```python
from build123d import *

# Parameters (mm, degrees)
BOSS_EXTRUDE1_DEPTH            = 60
CBORE_FOR_M3_SHCS1_D           = 3.4
CBORE_FOR_M3_SHCS1_DEPTH       = 5
CBORE_FOR_M3_SHCS1_CBORE_D     = 6.5
CBORE_FOR_M3_SHCS1_CBORE_DEPTH = 3
CBORE_FOR_M3_SHCS1_TIP         = 1.021463052


with BuildPart() as part:
    # Sketch3 → Boss-Extrude1 (new body)
    with BuildSketch(Plane.XY):
        Polygon((0, 60.2), (0, 33.96), (-3, 35.94), (-3, 55.2), (-12, 55.2), (-12, 60.2), align=None)
    extrude(amount=BOSS_EXTRUDE1_DEPTH)

    # CBORE for M3 SHCS1
    with Locations(Plane(origin=(0, 60.2, 0), x_dir=(1, 0, 0), z_dir=(0, 1, 0))):
        with Locations((-7.5, -15), (-7.5, -45)):
            CounterBoreHole(CBORE_FOR_M3_SHCS1_D / 2, CBORE_FOR_M3_SHCS1_CBORE_D / 2, CBORE_FOR_M3_SHCS1_CBORE_DEPTH, depth=CBORE_FOR_M3_SHCS1_DEPTH)
            with Locations((0, 0, -(CBORE_FOR_M3_SHCS1_DEPTH + CBORE_FOR_M3_SHCS1_TIP / 2))):  # 118° drill point
                Cone(0, CBORE_FOR_M3_SHCS1_D / 2, CBORE_FOR_M3_SHCS1_TIP, mode=Mode.SUBTRACT)


solid = part.part
```
Verification items for the finished model (mm, model axes). A direction names the side the tool comes from. Coordinates: 2 decimals unless noted, no trailing zeros. Loops run counter-clockwise (first coordinate to the right, second up) from the corner with the lowest first, then second, coordinate; pieces in that order, holes last. Notation, with made-up numbers: (6, 78) -> (42, 78) arc R31 ccw to (42, 111) -> close; hole circle Ø6 at (-18.5, 48). An arc over 180 degrees is marked (long way). Answer in a Markdown table with one row per item. Add a question column.
1. Section check A-A, the plane x = -7.5. Enter the section's corners in (y, z).
2. Depth check by flat-ended pin: P1, Ø1, axis at y = 40.5, z = 17, coming from the -X side; P2, Ø6, axis at x = -7.5, z = 45, coming from the +Y side; P3, Ø4, axis at x = -7.5, z = 15, coming from the -Y side. Enter the tip coordinate at first touch or a pass-through.
3. Access from +Z, -Z, +X, -X, +Y, -Y to the whole of each face (thin tool, end or side, straight path). Record for faces 1 (the face through (-6, 60.2, 30)), 2 (the face through (-6.1, 57.2, 16.4)), 3 (the face through (-7, 55.2, 30)).
4. Draft check along Z on faces 4 (the face through (-2, 53, 0)), 5 (the face through (-12, 58, 30)), 6 (the face through (-5.8, 56.19, 14.93)). Enter one of: +Z half, -Z half, draft (parallel to the pull), parting line (faces both ways), or undercut.
5. Section check D-D, the plane x = -1. Enter the section's corners in (y, z), then the cut area to 3 significant figures.
6. Material ranges on probe 1 along Z at (x, y) = (-7.5, 59.5); probe 2 along Z at (x, y) = (-7.5, 56.3); probe 3 along X at (y, z) = (55.65, 45), recorded low to high. Write a range as [from, to].
7. Section check C-C, the plane z = 36. Enter the section's corners in (x, y), then the cut area to 3 significant figures.
8. Section check B-B, the plane z = 45. Enter the section's corners in (x, y).
Derived:
| question | item | result |
|---|---|---|
| 1 | outline | (55.2, 0) -> (60.2, 0) -> (60.2, 11.75) -> (57.2, 11.75) -> (57.2, 13.3) -> (55.2, 13.3) -> close; (55.2, 16.7) -> (57.2, 16.7) -> (57.2, 18.25) -> (60.2, 18.25) -> (60.2, 41.75) -> (57.2, 41.75) -> (57.2, 43.3) -> (55.2, 43.3) -> close; (55.2, 46.7) -> (57.2, 46.7) -> (57.2, 48.25) -> (60.2, 48.25) -> (60.2, 60) -> (55.2, 60) -> close |
| 2 | P1 | stops at x = -3 |
| 2 | P2 | stops at y = 57.2 |
| 2 | P3 | stops at y = 55.2 |
| 3 | face 1 | +Z, -Z, +X, -X, +Y |
| 3 | face 2 | +Y |
| 3 | face 3 | +Z, -Z, -X, -Y |
| 4 | face 4 | -Z half |
| 4 | face 5 | draft |
| 4 | face 6 | undercut |
| 5 | outline | (34.62, 0) -> (60.2, 0) -> (60.2, 60) -> (34.62, 60) -> close |
| 5 | area | 1,530 mm² |
| 6 | probe 1 | z = [0, 11.75], [18.25, 41.75], [48.25, 60] |
| 6 | probe 2 | z = [0, 13.3], [16.7, 43.3], [46.7, 60] |
| 6 | probe 3 | x = [-12, -9.2], [-5.8, 0] |
| 7 | outline | (-12, 55.2) -> (-3, 55.2) -> (-3, 35.94) -> (0, 33.96) -> (0, 60.2) -> (-12, 60.2) -> close |
| 7 | area | 121 mm² |
| 8 | outline | (-12, 55.2) -> (-9.2, 55.2) -> (-9.2, 57.2) -> (-10.75, 57.2) -> (-10.75, 60.2) -> (-12, 60.2) -> close; (-5.8, 55.2) -> (-3, 55.2) -> (-3, 35.94) -> (0, 33.96) -> (0, 60.2) -> (-4.25, 60.2) -> (-4.25, 57.2) -> (-5.8, 57.2) -> close |
